Verification items for the finished model (mm, model axes). A direction names the side the tool comes from. Round coordinates to 2 decimals unless told otherwise and drop trailing zeros. Write each loop counter-clockwise with the first axis right and the second up, starting at its lowest first coordinate (ties: lowest second). Pieces come first, ordered by that corner, then holes. Notation, with made-up numbers: M 41.5,39 L 100.5,39 A28 cw 100.5,76 Z; hole C -24,3.25 d5. An arc over 180 degrees is marked long. One line per question, with ' | ' between items. Start each with the question number.
Q1. Cross-section at D-D (z = 53). Record the boundary of the cut face in (x, y).
Q2. Cross-section at C-C (z = 144.5). Record the boundary of the cut face in (x, y) (1 decimal).
Q3. Tool access check on faces 1 (the face through (4.3, 2.3, 0)), 2 (the face through (0, 0, 167)), 3 (the face through (4.3, 2.3, 86)). Record the directions out of +Z, -Z, +X, -X, +Y, -Y that give a thin tool (end or side, any length) a straight path to the whole face; none if there is none.
Q4. Thickness scan on line 1 along Z through (x, y) = (7.75, 4); line 2 along X through (y, z) = (-0.25, 54); line 3 along Y through (x, z) = (-2.25, 56.5). Record the ranges inside material, lowest first. Write a range as from..to.
Q5. Cross-section at A-A (y = 0). Record the boundary of the cut face in (x, z).
Q6. Gauge pin test, flat ends, axial feed: pin 1 (1 mm diameter, centred on x = 4, y = -7, fed in from -Z); pin 2 (3 mm diameter, centred on x = 5, y = -6, fed in from +Z); pin 3 (4 mm diameter, centred on x = 5, z = 128, fed in from +Y). Record the tip position at first contact, or that the pin passes through.
from build123d import *

# Parameters (mm, degrees)
SKETCH1_R                = 9.9
BOSS_EXTRUDE1_DEPTH      = 86
BOSS_EXTRUDE3_DEPTH      = 66
BOSS_EXTRUDE3_DEPTH_BACK = 97.65
SKETCH3_R                = 4.7125
BOSS_EXTRUDE2_START      = 66
SKETCH2_R                = 3
BOSS_EXTRUDE2_DEPTH      = 15


with BuildPart() as part:
    # Sketch1 → Boss-Extrude1 (new body)
    with BuildSketch(Plane.XY):
        Circle(SKETCH1_R)
    extrude(amount=BOSS_EXTRUDE1_DEPTH)

    # Sketch3 → Boss-Extrude3 (add, two sides: drawn at the far end of the back side and taken through both)
    with BuildSketch(Plane.XY.offset(86).offset(-BOSS_EXTRUDE3_DEPTH_BACK)):
        Circle(SKETCH3_R)
    extrude(amount=BOSS_EXTRUDE3_DEPTH + BOSS_EXTRUDE3_DEPTH_BACK)

    # Sketch2 → Boss-Extrude2 (add)
    with BuildSketch(Plane.XY.offset(86).offset(BOSS_EXTRUDE2_START)):
        Circle(SKETCH2_R)
    extrude(amount=BOSS_EXTRUDE2_DEPTH)


solid = part.part
Determined:
1) outline: C 0,0 d19.8
2) outline: C 0,0 d9.4
3) face 1: -Z | face 2: +Z, +X, -X, +Y, -Y | face 3: +Z
4) line 1: z = 0..86 | line 2: x = -9.9..9.9 | line 3: y = -9.64..9.64
5) outline: M -9.9,0 L -4.71,0 L -4.71,-11.65 L 4.71,-11.65 L 4.71,0 L 9.9,0 L 9.9,86 L 4.71,86 L 4.71,152 L 3,152 L 3,167 L -3,167 L -3,152 L -4.71,152 L -4.71,86 L -9.9,86 Z
6) pin 1: stops at z = 0 | pin 2: stops at z = 86 | pin 3: stops at y = 3.63
